Part model, mm, in its own coordinate system. Coordinates: 2 decimals unless noted, no trailing zeros. Loops run counter-clockwise (first coordinate to the right, second up) from the corner with the lowest first, then second, coordinate; pieces in that order, holes last.
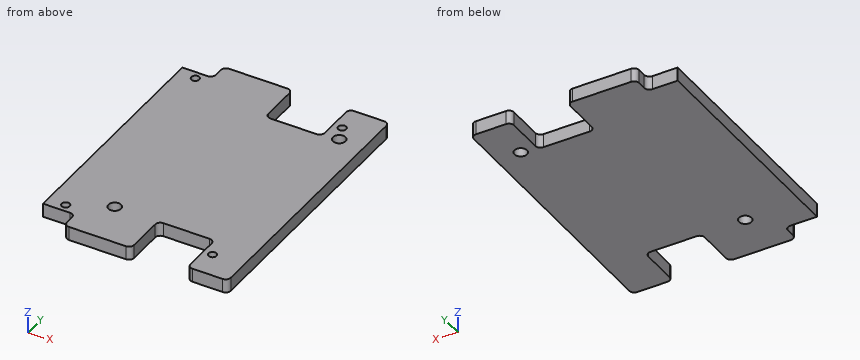
Autodesk Inventor part; units mm, degrees
ref_plane "YZ Plane" through (0, 0, 0) normal (1, 0, 0) x (0, 1, 0)
ref_plane "XZ Plane" through (0, 0, 0) normal (0, 1, 0) x (-1, 0, 0)
ref_plane "XY Plane" through (0, 0, 0) normal (0, 0, 1) x (1, 0, 0)
sketch "Sketch1" plane through (0, 0, 0) normal (0, 0, 1) x (1, 0, 0)
  line L0 (10.66, -31.5) -> (10.66, -19.9) construction
  line L1 (10.66, -31.5) -> (20, -31.5) construction
  line L2 (20, -31.5) -> (20, 31.5) construction
  line L3 (10.66, 31.5) -> (20, 31.5) construction
  line L4 (10.66, 19.9) -> (10.66, 31.5) construction
  arc A0 (9.66, 18.9) -> (10.66, 19.9) centre (9.66, 19.9) ccw construction
  line L5 (2.06, 18.9) -> (9.66, 18.9) construction
  arc A1 (1.06, 19.9) -> (2.06, 18.9) centre (2.06, 19.9) ccw construction
  line L6 (1.06, 31.5) -> (1.06, 19.9) construction
  line L7 (-20, 31.5) -> (1.06, 31.5) construction
  line L8 (-20, 31.5) -> (-20, -31.5) construction
  line L9 (-20, -31.5) -> (1.06, -31.5) construction
  line L10 (1.06, -19.9) -> (1.06, -31.5) construction
  arc A2 (2.06, -18.9) -> (1.06, -19.9) centre (2.06, -19.9) ccw construction
  line L11 (9.66, -18.9) -> (2.06, -18.9) construction
  arc A3 (10.66, -19.9) -> (9.66, -18.9) centre (9.66, -19.9) ccw construction
  line L12 (17.245, 17.9) -> (-18.765, 17.9) construction
  line L13 (17.245, -17.9) -> (17.245, 17.9) construction
  line L14 (-18.765, -17.9) -> (17.245, -17.9) construction
  line L15 (-18.765, 17.9) -> (-18.765, -17.9) construction
  circle A4 centre (0.9382, -13.2582) radius 1 construction
  circle A5 centre (-15.16, -21.5982) radius 1 construction
  circle A6 centre (-15.16, 21.6018) radius 1 construction
  circle A7 centre (13.64, 21.6018) radius 1 construction
  line L16 (10.84, 17.8518) -> (1.765, 17.8518)
  arc A8 (0.765, 18.8518) -> (1.765, 17.8518) centre (1.765, 18.8518) ccw
  line L17 (0.765, 26.467) -> (0.765, 18.8518)
  arc A9 (0.765, 26.467) -> (-0.06, 26.9018) centre (-0.06, 25.9018) ccw
  line L18 (-0.06, 26.9018) -> (-12.68, 26.9018)
  line L19 (-12.68, 26.9018) -> (-12.68, 24.2118)
  arc A10 (-13.68, 23.2118) -> (-12.68, 24.2118) centre (-13.68, 24.2118) ccw
  line L20 (-17.78, 23.2118) -> (-13.68, 23.2118)
  arc A11 (-18.78, 24.2118) -> (-17.78, 23.2118) centre (-17.78, 24.2118) ccw
  line L21 (-18.78, 26.9018) -> (-18.78, 24.2118)
  line L22 (-18.78, 26.9018) -> (-20.66, 26.9018)
  line L23 (-20.66, 26.9018) -> (-20.66, -26.8982)
  line L24 (-18.55, -26.8982) -> (-20.66, -26.8982)
  line L25 (-18.55, -26.8982) -> (-18.55, -24.2182)
  arc A12 (-17.55, -23.2182) -> (-18.55, -24.2182) centre (-17.55, -24.2182) ccw
  line L26 (-13.38, -23.2182) -> (-17.55, -23.2182)
  arc A13 (-12.38, -24.2182) -> (-13.38, -23.2182) centre (-13.38, -24.2182) ccw
  line L27 (-12.38, -26.8982) -> (-12.38, -24.2182)
  line L28 (-0.06, -26.8982) -> (-12.38, -26.8982)
  arc A14 (-0.06, -26.8982) -> (0.77, -26.4559) centre (-0.06, -25.8982) ccw
  line L29 (0.77, -26.4559) -> (0.77, -18.8482)
  arc A15 (1.77, -17.8482) -> (0.77, -18.8482) centre (1.77, -18.8482) ccw
  line L30 (1.77, -17.8482) -> (10.84, -17.8482)
  arc A16 (11.84, -18.8482) -> (10.84, -17.8482) centre (10.84, -18.8482) ccw
  line L31 (11.84, -18.8482) -> (11.84, -25.8982)
  arc A17 (11.84, -25.8982) -> (12.84, -26.8982) centre (12.84, -25.8982) ccw
  line L32 (17.74, -26.8982) -> (12.84, -26.8982)
  line L33 (17.74, -26.8982) -> (17.74, 26.9018)
  line L34 (17.74, 26.9018) -> (12.84, 26.9018)
  arc A18 (12.84, 26.9018) -> (11.84, 25.9018) centre (12.84, 25.9018) ccw
  line L35 (11.84, 25.9018) -> (11.84, 18.8518)
  arc A19 (10.84, 17.8518) -> (11.84, 18.8518) centre (10.84, 18.8518) ccw
  circle A20 centre (-15.16, 21.6018) radius 1
  circle A21 centre (-15.16, -21.5982) radius 1
  circle A22 centre (13.64, -21.5982) radius 1
  circle A23 centre (13.64, 21.6018) radius 1
  line L36 (-20.66, 0.0018) -> (17.74, 0.0018) construction
  line L37 (-1.46, 0.0018) -> (-1.46, -26.8982) construction
  line L38 (-20, 0) -> (20, 0) construction
  point P0 (-20.66, -26.8983)
  point P1 (17.64, 32.8018)
  dimension "d2" = 40
  dimension "d3" = 63
extrude "Extrusion1" add sketch "Sketch1" against normal blind 2.7 contours A19 L35 A18 L34 L33 L32 A17 L31 A16 L30 A15 L29 A14 L28 L27 A13 L26 A12 L25 L24 L23 L22 L21 A11 L20 A10 L19 L18 A9 L17 A8 L16 | A20 | A21 | A22 | A23
hole "Hole1" at (-15.16, -21.5982, 0) at (-15.16, 21.6018, 0) at (13.64, 21.6018, 0) at (13.64, -21.5982, 0) at (13.64, 21.6018, 0) at (-15.16, 21.6018, 0) at (-15.16, -21.5982, 0) direction (0, 0, -1) diameter 1.567 depth 2.5
sketch "Sketch2" plane through (0, 0, -2.7) normal (0, 0, -1) x (-1, 0, 0)
  circle A0 centre (-14.8923, 18.4994) radius 1.6002
  circle A1 centre (7.7497, -17.8506) radius 1.6002
  line L0 (-14.8923, 18.4994) -> (7.7497, 18.4994)
  line L1 (7.7497, 18.4994) -> (7.7497, -17.8506)
  line L2 (7.7497, -17.8506) -> (-14.8923, -17.8506)
  line L3 (-14.8923, -17.8506) -> (-14.8923, 18.4994)
hole "Hole2" at (-7.7497, -17.8506, -2.7) at (14.8923, 18.4994, -2.7) direction (0, 0, 1) diameter 2.459 end through all
sketch "Sketch4" plane through (0, 0, 0) normal (0, 0, 1) x (1, 0, 0)
  line L0 (-20.66, 26.9018) -> (-18.78, 26.9018)
  line L1 (-17.78, 23.2118) -> (-20.66, 23.2118)
  line L2 (-20.66, 23.2118) -> (-20.66, 26.9018)
  line L3 (-20.66, 26.9018) -> (-17.78, 26.9018)
  line L4 (-17.78, 26.9018) -> (-17.78, 23.2118)
  line L5 (-18.55, -26.8982) -> (-20.66, -26.8982)
  line L6 (-17.55, -23.2182) -> (-20.66, -23.2182)
  line L7 (-20.66, -23.2182) -> (-20.66, -26.8982)
  line L8 (-20.66, -26.8982) -> (-17.55, -26.8982)
  line L9 (-17.55, -26.8982) -> (-17.55, -23.2182)
  point P0 (0, 0)
extrude "Extrusion4" cut sketch "Sketch4" against normal blind 10
sketch "Sketch5" plane through (-20.66, -23.2182, 0) normal (-1, 0, 0) x (0, 0, 1)
  line L0 (0, 46.43) -> (-2.7, 46.43)
  line L1 (-2.7, 0) -> (-2.7, 46.43)
  line L2 (-2.7, 0) -> (0, 0)
  line L3 (0, 46.43) -> (0, 0)
  point P0 (0, 23.2182)
extrude "Extrusion5" cut sketch "Sketch5" against normal blind 2
sketch "Sketch6" plane through (17.74, -26.8982, 0) normal (1, 0, 0) x (0, 0, -1)
  line L0 (0, 0) -> (0, 53.8)
  line L1 (0, 0) -> (2.7, 0)
  line L2 (2.7, 53.8) -> (2.7, 0)
  line L3 (0, 53.8) -> (2.7, 53.8)
  point P0 (0, 26.8982)
extrude "Extrusion6" add sketch "Sketch6" along normal blind 2
sketch "Sketch7" plane through (0, 0, -2.7) normal (0, 0, -1) x (-1, 0, 0)
  arc A0 (-0.77, -26.4559) -> (0.06, -26.8982) centre (0.06, -25.8982) ccw
  line L0 (-0.77, -26.4559) -> (0.06, -26.4559)
  line L1 (0.06, -26.4559) -> (0.06, -26.8982)
  line L2 (0.06, -26.8982) -> (-0.77, -26.8982)
  line L3 (-0.77, -26.8982) -> (-0.77, -26.4559)
  arc A1 (0.06, 26.9018) -> (-0.765, 26.467) centre (0.06, 25.9018) ccw
  line L4 (0.06, 26.9018) -> (-0.765, 26.9018)
  line L5 (-0.765, 26.9018) -> (-0.765, 26.467)
  line L6 (-0.765, 26.467) -> (0.06, 26.467)
  line L7 (0.06, 26.467) -> (0.06, 26.9018)
  point P0 (0, 0)
extrude "Extrusion7" add sketch "Sketch7" against normal up to surface (2.7 mm away)
fillet "Fillet3" radius 1 6 edges at (-12.38, -26.8982, -1.35) (19.74, -26.8982, -1.35) (19.74, 26.9018, -1.35) (-12.68, 26.9018, -1.35) (0.765, 26.9018, -1.35) (0.77, -26.8982, -1.35)
properties part number "3d_LM - chapa" material "Aluminium 6061-T6"
Q1. Saw through at A-A (x = -15.16). List the corners of the cut face in (y, z), plus the area to 3 significant figures.
Q2. Saw through at D-D (z = -0.45). Count the separate pieces of the cut face and the enclosed holes in it, plus the area to 3 significant figures.
Q3. Probe line 1 (Y direction, x = 15, z = -1.3); line 2 (X direction, y = -20.5, z = -2.4); line 3 (X direction, y = -23.5, z = -1.95). List the from-to ranges inside material, lowest first.
Q4. Drop flat-ended pins along their axis: P1, Ø1.4, axis at x = 7.5, z = -1, coming from the -Y side; P2, Ø0.8, axis at x = -17, z = -1, coming from the +Y side. Give the stop position or say it passes through.
Q5. Saw through at C-C (x = 15.5). List the corners of the cut face in (y, z), plus the area to 3 significant figures.
Q6. Saw through at B-B (y = 21.5). List the corners of the cut face in (x, z) (3 decimals), plus the area to 3 significant figures.
Checked values:
1. outline: (-23.22, -2.7) - (23.21, -2.7) - (23.21, 0) - (22.39, 0) - (22.39, -2.5) - (20.82, -2.5) - (20.82, 0) - (-20.81, 0) - (-20.81, -2.5) - (-22.38, -2.5) - (-22.38, 0) - (-23.22, 0) - close
1. area: 118 mm2
2. separate pieces: 1
2. enclosed holes: 6
2. area: 1,800 mm2
3. line 1: y = -26.9 to 17.27, 19.72 to 26.9
3. line 2: x = -18.66 to 0.77, 11.84 to 19.74
3. line 3: x = -12.68 to 0.77, 11.84 to 19.74
4. P1: stops at y = -17.85
4. P2: stops at y = 23.21
5. outline: (-26.9, -2.7) - (17.43, -2.7) - (17.43, 0) - (-26.9, 0) - close; (19.57, -2.7) - (26.9, -2.7) - (26.9, 0) - (19.57, 0) - close
5. area: 139 mm2
6. outline: (-18.66, -2.7) - (0.765, -2.7) - (0.765, 0) - (-14.383, 0) - (-14.383, -2.5) - (-15.937, -2.5) - (-15.937, 0) - (-18.66, 0) - close; (11.84, -2.7) - (19.74, -2.7) - (19.74, 0) - (14.417, 0) - (14.417, -2.5) - (12.863, -2.5) - (12.863, 0) - (11.84, 0) - close
6. area: 66.0 mm2
